```python
from build123d import *

# Parameters (mm, degrees)
SKETCH2_R           = 2
SKETCH2_R_2         = 1.999999991
BOSS_EXTRUDE1_DEPTH = 5.588
SKETCH7_R           = 2.032
CUT_EXTRUDE1_DEPTH  = 5.588


with BuildPart() as part:
    # Sketch2 → Boss-Extrude1 (new body)
    with BuildSketch(Plane(origin=(0, 0, 0), x_dir=(1, 0, 0), z_dir=(0, 1, 0))):
        with BuildLine():
            ThreePointArc((17.295902343, -30.526810701), (16.688093876, -28.878103365), (15.15555913, -28.018449791))
            Line((15.15555913, -28.018449791), (13.238676936, -27.713033224))
            ThreePointArc((13.238676936, -27.713033224), (11.241051513, -26.538356195), (10.573787778, -24.319092227))
            Line((10.573787778, -24.319092227), (12.5603, 0))
            ThreePointArc((12.5603, 0), (0.603657177, 12.545785512), (-12.502275592, 1.2059192))
            Line((-12.502275592, 1.2059192), (-16.498266045, -40.222207921))
            ThreePointArc((-16.498266045, -40.222207921), (-16.507064815, -40.344000039), (-16.51, -40.466074291))
            Line((-16.51, -40.466074291), (-16.51, -221.328861788))
            ThreePointArc((-16.51, -221.328861788), (-12.970187584, -225.680718913), (-7.988667969, -223.101301399))
            Line((-7.988667969, -223.101301399), (16.979901226, -165.677523619))
            ThreePointArc((16.979901226, -165.677523619), (17.216065593, -164.934164738), (17.295902343, -164.158289667))
            Line((17.295902343, -164.158289667), (17.295902343, -30.526810701))
        make_face()
        with Locations((-11.43, -219.075)):
            Circle(SKETCH2_R, mode=Mode.SUBTRACT)
        with Locations((-11.43, -212.725)):
            Circle(SKETCH2_R, mode=Mode.SUBTRACT)
        with Locations((-11.43, -206.375)):
            Circle(SKETCH2_R, mode=Mode.SUBTRACT)
        with Locations((-11.43, -200.025)):
            Circle(SKETCH2_R, mode=Mode.SUBTRACT)
        with BuildLine():
            ThreePointArc((7.135902343, -162.410770806), (8.023611961, -165.648962244), (10.438542905, -167.981776143))
            Line((10.438542905, -167.981776143), (-0.534170778, -193.217289931))
            ThreePointArc((-0.534170778, -193.217289931), (-2.234040931, -194.665234867), (-4.420389569, -194.211381682))
            Line((-4.420389569, -194.211381682), (-11.716886202, -188.551043102))
            ThreePointArc((-11.716886202, -188.551043102), (-12.441018517, -187.661516081), (-12.7, -186.544128716))
            Line((-12.7, -186.544128716), (-12.7, -149.615408258))
            ThreePointArc((-12.7, -149.615408258), (-11.988693683, -148.474898999), (-10.651556899, -148.611951065))
            Line((-10.651556899, -148.611951065), (7.135902343, -162.410770806))
        make_face(mode=Mode.SUBTRACT)
        with BuildLine():
            ThreePointArc((10.656105825, -153.315833936), (9.771695946, -153.639779081), (8.923603828, -154.049487576))
            Line((8.923603828, -154.049487576), (-10.733772403, -138.80005889))
            ThreePointArc((-10.733772403, -138.80005889), (-12.182037035, -137.021004847), (-12.7, -134.786230117))
            Line((-12.7, -134.786230117), (-12.7, -90.4875))
            ThreePointArc((-12.7, -90.4875), (-11.803536501, -90.43671411), (-10.918544548, -90.285006317))
            Line((-10.918544548, -90.285006317), (10.027134635, -128.362607876))
            ThreePointArc((10.027134635, -128.362607876), (10.49635106, -129.547067395), (10.656105825, -130.811024207))
            Line((10.656105825, -130.811024207), (10.656105825, -153.315833936))
        make_face(mode=Mode.SUBTRACT)
        with Locations((13.485902343, -162.410770806)):
            Circle(SKETCH2_R, mode=Mode.SUBTRACT)
        with BuildLine():
            Line((-10.16, -44.337182032), (1.663048834, -44.337182032))
            ThreePointArc((1.663048834, -44.337182032), (2.739129831, -44.932682449), (2.806066447, -46.160725831))
            Line((2.806066447, -46.160725831), (-11.055993219, -74.784618621))
            ThreePointArc((-11.055993219, -74.784618621), (-11.873503915, -74.655646925), (-12.7, -74.6125))
            Line((-12.7, -74.6125), (-12.7, -46.877182032))
            ThreePointArc((-12.7, -46.877182032), (-11.956051224, -45.081130808), (-10.16, -44.337182032))
        make_face(mode=Mode.SUBTRACT)
        with BuildLine():
            ThreePointArc((-9.903213406, -40.527182032), (-11.783508673, -39.694838236), (-12.431479451, -37.743315662))
            Line((-12.431479451, -37.743315662), (-9.755434212, -9.99962016))
            ThreePointArc((-9.755434212, -9.99962016), (-2.756273581, -13.695395429), (5.127655889, -12.99492382))
            Line((5.127655889, -12.99492382), (3.069264048, -38.19397392))
            ThreePointArc((3.069264048, -38.19397392), (2.259083254, -39.854914801), (0.537695935, -40.527182032))
            Line((0.537695935, -40.527182032), (-9.903213406, -40.527182032))
        make_face(mode=Mode.SUBTRACT)
        with BuildLine():
            Line((-3.521718331, 2), (3.521718331, 2))
            ThreePointArc((3.521718331, 2), (0, -4.05), (-3.521718331, 2))
        make_face(mode=Mode.SUBTRACT)
        with BuildLine():
            ThreePointArc((-8.804706991, -86.222769023), (-8.262040897, -82.55), (-8.804706991, -78.877230977))
            Line((-8.804706991, -78.877230977), (7.575478058, -45.053638233))
            ThreePointArc((7.575478058, -45.053638233), (8.043996088, -44.531101035), (8.718495671, -44.337182032))
            Line((8.718495671, -44.337182032), (10.945902343, -44.337182032))
            ThreePointArc((10.945902343, -44.337182032), (11.843927955, -44.70915642), (12.215902343, -45.607182032))
            Line((12.215902343, -45.607182032), (12.215902343, -62.618124667))
            ThreePointArc((12.215902343, -62.618124667), (6.881902343, -71.709053992), (12.215902343, -80.799983318))
            Line((12.215902343, -80.799983318), (12.215902343, -119.492817968))
            ThreePointArc((12.215902343, -119.492817968), (11.261891546, -120.722879277), (9.83314514, -120.104922051))
            Line((9.83314514, -120.104922051), (-8.804706991, -86.222769023))
        make_face(mode=Mode.SUBTRACT)
        with Locations((13.485902343, -38.1)):
            Circle(SKETCH2_R_2, mode=Mode.SUBTRACT)
    extrude(amount=BOSS_EXTRUDE1_DEPTH)

    # Sketch7 → Cut-Extrude1 (cut)
    with BuildSketch(Plane(origin=(0, 5.588, 0), x_dir=(1, 0, 0), z_dir=(0, 1, 0))):
        with Locations((12.215902343, -71.655983318)):
            Circle(SKETCH7_R)
    extrude(amount=-CUT_EXTRUDE1_DEPTH, mode=Mode.SUBTRACT)


solid = part.part
```
Geometry check sheet. Reference: the model listing, model coordinates, mm. A direction names the side the tool comes from. Round coordinates to 2 decimals unless told otherwise and drop trailing zeros. Order: outer loops, then holes, each group sorted by start corner. A loop starts at its lowest first (then second) coordinate and runs counter-clockwise, first axis right, second up. Notation, with made-up numbers: M 12,86 L 35,86 A36 ccw 35,123 Z; hole C -16.75,71.25 d3. An arc over 180 degrees is marked long. Write item = value, one per line.
Q1. Section check B-B (z = 65.5). Enter the section's corners in (x, y), plus the area to 3 significant figures.
Answer block:
outline = M -16.51,0 L -12.7,0 L -12.7,5.59 L -16.51,5.59 Z; M -6.56,0 L -2.33,0 L -2.33,5.59 L -6.56,5.59 Z; M 8.94,0 L 17.3,0 L 17.3,5.59 L 8.94,5.59 Z
area = 91.7 mm^2
Q2. Section check C-C (y = 3.75). Give the number of separate pieces and of enclosed holes in the cut face, plus the area to 3 significant figures.
Answer block:
separate_pieces = 1
enclosed_holes = 13
area = 3,510 mm^2
Q3. Set-up check for faces 4 (the flat face through (0, 5.588, 105)), 5 (the cylindrical face through (-8.262, 2.755, 82.602)): record each of +Z, -Z, +X, -X, +Y, -Y from which the full face is reachable in a straight line by a thin tool's end or side.
Answer block:
face_4 = +Z, -Z, +X, -X, +Y
face_5 = +Y, -Y
Q4. Scan lines: line 1 (Z direction, x = 9.5, y = 2.2); line 2 (X direction, y = 1.85, z = 38.1); line 3 (X direction, y = 4.05, z = 57). Record each from-to range of solid material in increasing order.
Answer block:
line_1 = -8.22 to 44.34, 64.8 to 78.61, 119.5 to 127.4, 153.76 to 167.35, 170.14 to 182.88
line_2 = -16.29 to -12.44, 3.08 to 11.49, 15.49 to 17.3
line_3 = -16.51 to -12.7, -2.44 to 1.79, 12.22 to 17.3
Q5. Depth check by flat-ended pin: pin 1 Ø0.7 at (x, y) = (10.5, 2.5) entering from +Z; pin 2 Ø3 at (x, y) = (3.5, 2.5) entering from -Z; pin 3 Ø1 at (x, y) = (-10, 4) entering from +Z; pin 4 Ø10.5 at (x, z) = (0, 0) entering from +Y. Enter the tip coordinate at first touch or a pass-through.
Answer block:
pin_1 = 181.39
pin_2 = -12.4
pin_3 = 225.49
pin_4 = 5.59
Q6. Section check D-D (z = 95.5). Enter the section's corners in (x, y).
Answer block:
outline = M -16.51,0 L -12.7,0 L -12.7,5.59 L -16.51,5.59 Z; M -8.05,0 L -3.7,0 L -3.7,5.59 L -8.05,5.59 Z; M 12.22,0 L 17.3,0 L 17.3,5.59 L 12.22,5.59 Z
Q7. Release check for a two-part mould opening along X. For faces 1 (the flat face through (-8.02, 2.75, 191.42)), 2 (the flat face through (11.553, 2.755, 12.33)), 3 (the flat face through (-16.51, 3, 130)) record: released by +X, released by -X, zero draft, split by the parting line, or undercut.
Answer block:
face_1 = undercut
face_2 = released by +X
face_3 = released by -X
Q8. Section check A-A (z = 158). Enter the section's corners in (x, y).
Answer block:
outline = M -16.51,0 L -12.7,0 L -12.7,5.59 L -16.51,5.59 Z; M 1.45,0 L 17.3,0 L 17.3,5.59 L 1.45,5.59 Z
